Autodesk Fusion 360 part; units mm, degrees
sketch "Sketch1" plane through (0, 0, 0) normal (0, 0, 1) x (1, 0, 0)
  circle A0 centre (0, 0) radius 38.0746
  dimension "d1" = 76.1492
extrude "Extrude1" add sketch "Sketch1" along normal blind 3.175
sketch "Sketch2" plane through (0, 0, 3.175) normal (0, 0, 1) x (-1, 0, 0)
  circle A0 centre (0, 0) radius 38.0746
  circle A1 centre (0, 0) radius 36.5125
  dimension "d4" = 73.025
extrude "Extrude2" add sketch "Sketch2" along normal blind 3.175 contours A1
sketch "Sketch3" plane through (0, 0, 6.35) normal (0, 0, 1) x (-1, 0, 0)
  circle A0 centre (0, 0) radius 36.5125
  circle A1 centre (25.4, -7.62) radius 3.175
  circle A2 centre (-25.4, -7.62) radius 3.175
  circle A3 centre (0, 20.6756) radius 5.08
  circle A4 centre (0, 0) radius 38.0746
  dimension "d7" = 50.8
  dimension "d8" = 25.4
  dimension "d9" = 7.62
  dimension "d10" = 6.35
  dimension "d11" = 6.35
  dimension "d12" = 10.16
  dimension "d13" = 20.6756
extrude "Extrude3" cut sketch "Sketch3" against normal blind 6.35 contours A1 | A2 | A3
equation "d2 = ( 0.25 / 2 ) * 1 in"
equation "d5 = ( 0.25 / 2 ) * 1 in"
Design review of the part built by this model. Coordinates are the model's own, in mm. A direction names the side the tool comes from. Round coordinates to 2 decimals unless told otherwise and drop trailing zeros. Write each loop counter-clockwise with the first axis right and the second up, starting at its lowest first coordinate (ties: lowest second). Pieces come first, ordered by that corner, then holes. Notation, with made-up numbers: M -28.5,44 L 23.5,44 A34 ccw 23.5,83 Z; hole C 67.25,31.5 d8. An arc over 180 degrees is marked long. One line per item, written item: value. Start each with the question number.
1. Take a section at C-C on y = 7.62. State the section outline as (x, z) points (3 decimals), then the cut area to 3 significant figures.
2. To check wall thickness, follow probe 1 along X at (y, z) = (7.62, 4.25) (3 decimals); probe 2 along X at (y, z) = (6.5, 1.5); probe 3 along Y at (x, z) = (0, 1.75). State the ranges of each line that lie inside material, in increasing order. Write a range as from..to.
3. For faces 4 (the face through (22.37, 6.67, 3.22)), 5 (the face through (-34.826, 10.967, 4.74)), list the 3-axis set-ups (+Z, -Z, +X, -X, +Y, -Y) from which the entire face can be reached by the end or side of a thin tool; tool diameter is ignored.
4. Take a section at D-D on y = -24.5. State the section outline as (x, z) points (3 decimals), then the cut area to 3 significant figures.
5. Draft analysis for pull direction Y (two halves, no side actions). For faces 1 (the face through (31, -20, 3.175)), 2 (the face through (36.316, -11.437, 1.565)), 3 (the face through (-28.43, 6.67, 3.22)), state which applies: pulls with the +Y half, pulls with the -Y half, needs draft (parallel to the pull), parting line crosses it, or undercut.
6. Clearance check with flat-ended pins moving along their axes: P1, Ø8, axis at x = 0, y = -20.68, coming from the -Z side; P2, Ø2, axis at x = -28, z = 4, coming from the -Y side; P3, Ø1, axis at x = -21.5, z = 4.5, coming from the -Y side; P4, Ø1, axis at y = 19.5, z = 1.5, coming from the -X side. State where each tip first meets the part, or that it passes through.
7. Take a section at A-A on x = -25.4. State the section outline as (y, z) points (3 decimals), then the cut area to 3 significant figures.
Computed:
1. outline: M -37.304,0 L -28.575,0 L -28.575,6.35 L -35.709,6.35 L -35.709,3.175 L -37.304,3.175 Z; M -22.225,0 L 22.225,0 L 22.225,6.35 L -22.225,6.35 Z; M 28.575,0 L 37.304,0 L 37.304,3.175 L 35.709,3.175 L 35.709,6.35 L 28.575,6.35 Z
1. area: 383 mm²
2. probe 1: x = -35.709..-28.575, -22.225..22.225, 28.575..35.709
2. probe 2: x = -37.52..-28.37, -22.43..22.43, 28.37..37.52
2. probe 3: y = -38.07..-25.76, -15.6..38.07
3. face 4: +Z, -Z
3. face 5: +Z
4. outline: M -29.145,0 L -3.344,0 L -3.344,6.35 L -27.072,6.35 L -27.072,3.175 L -29.145,3.175 Z; M 3.344,0 L 29.145,0 L 29.145,3.175 L 27.072,3.175 L 27.072,6.35 L 3.344,6.35 Z
4. area: 315 mm²
5. face 1: needs draft
5. face 2: parting line crosses it
5. face 3: undercut
6. P1: passes through
6. P2: stops at y = -26.4
6. P3: stops at y = -29.87
6. P4: stops at x = -33
7. outline: M -28.364,0 L 4.445,0 L 4.445,6.35 L -26.23,6.35 L -26.23,3.175 L -28.364,3.175 Z; M 10.795,0 L 28.364,0 L 28.364,3.175 L 26.23,3.175 L 26.23,6.35 L 10.795,6.35 Z
7. area: 306 mm²
